from build123d import *

# Parameters (mm, degrees)
CROQUIS1_W              = 50.4
CROQUIS1_H              = 73
SALIENTE_EXTRUIR1_DEPTH = 1
CROQUIS2_W              = 47.2
CROQUIS2_H              = 69.8
CORTAR_EXTRUIR1_DEPTH   = 0.4
CROQUIS3_W              = 11.5
CROQUIS3_H              = 1.6
CORTAR_EXTRUIR2_DEPTH   = 0.9


with BuildPart() as part:
    # Croquis1 → Saliente-Extruir1 (new body)
    with BuildSketch(Plane.XY):
        Rectangle(CROQUIS1_W, CROQUIS1_H)
    extrude(amount=SALIENTE_EXTRUIR1_DEPTH)

    # Croquis2 → Cortar-Extruir1 (cut)
    with BuildSketch(Plane.XY.offset(1)):
        Rectangle(CROQUIS2_W, CROQUIS2_H)
    extrude(amount=-CORTAR_EXTRUIR1_DEPTH, mode=Mode.SUBTRACT)

    # Croquis3 → Cortar-Extruir2 (cut)
    with BuildSketch(Plane.XY.offset(1.6)):
        with Locations((0.05, -35.7)):
            Rectangle(CROQUIS3_W, CROQUIS3_H)
    extrude(amount=-CORTAR_EXTRUIR2_DEPTH, mode=Mode.SUBTRACT)


solid = part.part
Geometry check sheet. Reference: the model listing, model coordinates, mm. A direction names the side the tool comes from. Give positions to 0.01 mm unless a question says otherwise; leave off trailing zeros. Order: outer loops, then holes, each group sorted by start corner. A loop starts at its lowest first (then second) coordinate and runs counter-clockwise, first axis right, second up.
1. Sectioned sample at B-B (x = -17). Record the boundary of the cut face in (y, z), then the cut area to 3 significant figures.
Completed:
outline: (-36.5, 0) - (36.5, 0) - (36.5, 1) - (34.9, 1) - (34.9, 0.6) - (-34.9, 0.6) - (-34.9, 1) - (-36.5, 1) - close
area: 45.1 mm2
2. Draft check along Y on faces 3 (the face through (-24, 0, 1)), 4 (the face through (0, 0, 0.6)). Enter one of: pulls with the +Y half, pulls with the -Y half, needs draft (parallel to the pull), parting line crosses it, or undercut.
Completed:
face 3: needs draft
face 4: undercut
3. Depth check by flat-ended pin: pin 1 (23.5 mm diameter, centred on x = -9.5, y = -6, fed in from +Z); pin 2 (0.5 mm diameter, centred on x = -3, y = -36, fed in from +Z). Enter the tip coordinate at first touch or a pass-through.
Completed:
pin 1: stops at z = 0.6
pin 2: stops at z = 0.7
4. Scan lines: line 1 (Y direction, x = 21.5, z = 0.85); line 2 (X direction, y = 16.5, z = 0.75); line 3 (Z direction, x = 20, y = 16.5). Record each from-to range of solid material in increasing order.
Completed:
line 1: y = -36.5 to -34.9, 34.9 to 36.5
line 2: x = -25.2 to -23.6, 23.6 to 25.2
line 3: z = 0 to 0.6
5. Sectioned sample at A-A (y = -14). Record the boundary of the cut face in (x, z).
Completed:
outline: (-25.2, 0) - (25.2, 0) - (25.2, 1) - (23.6, 1) - (23.6, 0.6) - (-23.6, 0.6) - (-23.6, 1) - (-25.2, 1) - close
6. Access from +Z, -Z, +X, -X, +Y, -Y to the whole of each face (thin tool, end or side, straight path). Record for faces 1 (the face through (0, -36, 0.7)), 2 (the face through (0, 1, 0)).
Completed:
face 1: +Z, -Y
face 2: -Z, +X, -X, +Y, -Y
